from build123d import *

# Parameters (mm, degrees)
BOSS_EXTRUDE1_DEPTH = 9
FILLET1_R           = 6
FILLET2_R           = 4
BOSS_EXTRUDE2_DEPTH = 18
LPATTERN1_COUNT     = 6
LPATTERN1_PITCH     = 6
CUT_EXTRUDE1_DEPTH  = 26
CUT_EXTRUDE3_DEPTH  = 10
SKETCH5_R           = 1.5
CUT_EXTRUDE4_DEPTH  = 124.909348227
SKETCH6_R           = 1.75
BOSS_EXTRUDE3_DEPTH = 3
SKETCH7_R           = 1.25
CUT_EXTRUDE6_DEPTH  = 1
SKETCH8_R           = 1.25
CUT_EXTRUDE7_DEPTH  = 1
CUT_EXTRUDE8_DEPTH  = 1


with BuildPart() as part:
    # Sketch1 → Boss-Extrude1 (new, symmetric)
    with BuildSketch(Plane(origin=(0, 0, 0), x_dir=(1, 0, 0), z_dir=(0, 1, 0))):
        with BuildLine():
            ThreePointArc((13.432245527, -50.487906924), (21.509028276, -53.088979862), (18.907955338, -61.165762611))
            Line((18.907955338, -61.165762611), (11, -67.286566673))
            Line((11, -67.286566673), (11, -117.286566673))
            Line((11, -117.286566673), (0, -117.286566673))
            Line((0, -117.286566673), (0, -110.286566673))
            Line((0, -110.286566673), (-20.129396013, -88.042299634))
            Line((-20.129396013, -88.042299634), (-31.928362438, -82.58479184))
            Line((-31.928362438, -82.58479184), (-27.730279519, -73.508663821))
            Line((-27.730279519, -73.508663821), (-24.896421124, -73.027946621))
            Line((-24.896421124, -73.027946621), (-12.941547125, -71))
            Line((-12.941547125, -71), (-4.10711559, -69.126148868))
            Line((-4.10711559, -69.126148868), (13.432245527, -50.487906924))
        make_face()
        Polygon((-12.941547125, -71), (-24.896421124, -73.027946621), (-36.603518956, -4.013862114), (-12.941547125, 0), align=None)
    extrude(amount=BOSS_EXTRUDE1_DEPTH, both=True)

    # Fillet1
    fillet1_edges = [part.edges().sort_by_distance(p)[0] for p in [
        (-36.603518956, 0, 4.013862114),
        (-12.941547125, 0, 0),
    ]]
    fillet(fillet1_edges, radius=FILLET1_R)

    # Fillet2
    fillet2_edges = [part.edges().sort_by_distance(p)[0] for p in [
        (0, 0, 117.286566673),
        (-31.928362438, 0, 82.58479184),
        (-27.730279519, 0, 73.508663821),
    ]]
    fillet(fillet2_edges, radius=FILLET2_R)

    # Sketch2 → Boss-Extrude2 (add)
    with BuildSketch(Plane(origin=(0, 9, 0), x_dir=(1, 0, 0), z_dir=(0, 1, 0))):
        Polygon((15, -112.286566673), (11, -114.265571656), (11, -110.265571656), align=None)
    boss_extrude2 = extrude(amount=-BOSS_EXTRUDE2_DEPTH)

    # LPattern1: Boss-Extrude2 ×6
    with Locations(*[(0, 0, -i * LPATTERN1_PITCH) for i in range(1, LPATTERN1_COUNT)]):
        add(boss_extrude2)

    # Sketch3 → Cut-Extrude1 (cut)
    with BuildSketch(Plane(origin=(0, 9, 0), x_dir=(1, 0, 0), z_dir=(0, 1, 0))):
        Polygon((8.082911966, -112.457569416), (8.082911966, -87.457569416), (-6.917088034, -87.457569416), align=None)
    extrude(amount=-CUT_EXTRUDE1_DEPTH, mode=Mode.SUBTRACT)

    # Sketch4 → Cut-Extrude3 (cut)
    with BuildSketch(Plane(origin=(-54.869240858, 0, 49.65255435), x_dir=(0.6709798671072843, 0, 0.7414755679971466), z_dir=(-0.7414755679971466, 0, 0.6709798671072843))):
        Polygon((60.774794667, 6), (60.774794667, -6), (78.951118156, -8.019187605), (78.951118156, 8.019187605), align=None)
    extrude(amount=-CUT_EXTRUDE3_DEPTH, mode=Mode.SUBTRACT)

    # Sketch5 → Cut-Extrude4 (cut, through all)
    with BuildSketch(Plane(origin=(0, 9, 0), x_dir=(1, 0, 0), z_dir=(0, 1, 0))):
        with Locations(Location((-29.68456047, -8.925889543, 0), (0, 0, 270))):
            Circle(SKETCH5_R)
    extrude(amount=-CUT_EXTRUDE4_DEPTH, mode=Mode.SUBTRACT)

    # Sketch6 → Boss-Extrude3 (add)
    with BuildSketch(Plane(origin=(0, 9, 0), x_dir=(1, 0, 0), z_dir=(0, 1, 0))):
        with Locations(Location((-26.618678063, -80.6335738, 0), (0, 0, 270))):
            Circle(SKETCH6_R)
        with Locations(Location((16.170100432, -55.826834767, 0), (0, 0, 270))):
            Circle(SKETCH6_R)
    boss_extrude3 = extrude(amount=BOSS_EXTRUDE3_DEPTH)

    # Sketch7 → Cut-Extrude6 (cut)
    with BuildSketch(Plane(origin=(0, 12, 0), x_dir=(1, 0, 0), z_dir=(0, 1, 0))):
        with Locations(Location((-26.618678063, -80.6335738, 0), (0, 0, 270))):
            Circle(SKETCH7_R)
    extrude(amount=-CUT_EXTRUDE6_DEPTH, mode=Mode.SUBTRACT)

    # Sketch8 → Cut-Extrude7 (cut)
    with BuildSketch(Plane(origin=(0, 12, 0), x_dir=(1, 0, 0), z_dir=(0, 1, 0))):
        with Locations(Location((16.170100432, -55.826834767, 0), (0, 0, 270))):
            Circle(SKETCH8_R)
    extrude(amount=-CUT_EXTRUDE7_DEPTH, mode=Mode.SUBTRACT)

    # Sketch9 → Cut-Extrude8 (cut)
    with BuildSketch(Plane(origin=(0, 9, 0), x_dir=(1, 0, 0), z_dir=(0, 1, 0))):
        with BuildLine():
            Line((-25.196199852, -15.539852581), (-16.757464085, -65.251677823))
            ThreePointArc((-16.757464085, -65.251677823), (-19.027845143, -68.450467492), (-22.226634811, -66.180086434))
            Line((-22.226634811, -66.180086434), (-30.665370577, -16.468261192))
            ThreePointArc((-30.665370577, -16.468261192), (-28.39498952, -13.269471524), (-25.196199852, -15.539852581))
        make_face()
    cut_extrude8 = extrude(amount=-CUT_EXTRUDE8_DEPTH, mode=Mode.SUBTRACT)

    # Mirror1: Boss-Extrude3, Cut-Extrude8 across plane
    add(boss_extrude3.mirror(Plane.ZX))
    add(cut_extrude8.mirror(Plane.ZX), mode=Mode.SUBTRACT)


solid = part.part
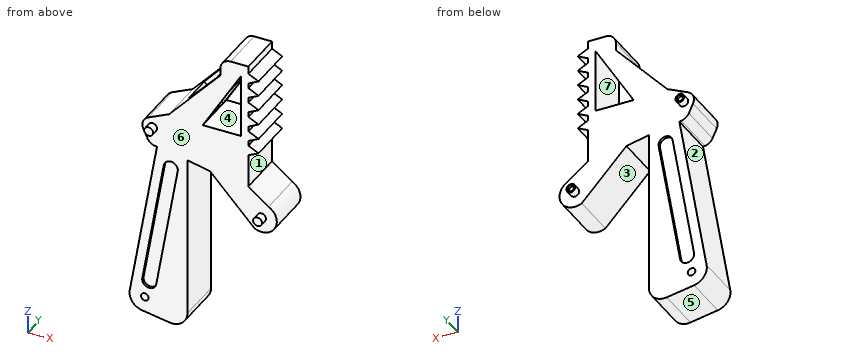
Model file for the job. Use its own axes, mm. Face numbers are marked on the shaded views. A direction names the side the tool comes from. Round coordinates to 2 decimals unless told otherwise and drop trailing zeros. Loops run counter-clockwise (first coordinate to the right, second up) from the corner with the lowest first, then second, coordinate; pieces in that order, holes last. Notation, with made-up numbers: (26.5, 63.25) -> (37.5, 63.25) arc R7 cw to (37.5, 73.25) -> close; hole circle Ø2 at (2.25, 56.25). An arc over 180 degrees is marked (long way). Answer as CSV lines item,"result". Start each with the question number.
1) Slice it at C-C (y = -10.25). List the corners of the cut face in (x, z), plus the area to 3 significant figures.
2) Probe line 1 along X through (y, z) = (8.5, 48); line 2 along Z through (x, y) = (7, 2.5); line 3 along Y through (x, z) = (-15.5, 22). List the from-to ranges inside material, lowest first.
3) Pin check, flat tips, straight feed: P1, Ø7.5, axis at x = -0.5, y = -4.5, coming from the +Z side; P2, Ø3, axis at x = -4, z = 87.5, coming from the +Y side; P3, Ø0.8, axis at x = -26.5, z = 81, coming from the +Y side. Stop position of each tip, or through.
4) Slice it at D-D (x = -11.5). List the corners of the cut face in (y, z).
5) Tool access for the marked faces 1, 2 and 3: list every direction of +Z, -Z, +X, -X, +Y, -Y with a clear straight run to the whole face (end or side of a thin tool).
6) Mould opens along X. For the marked faces 4, 5, 6 and 7 say: +X half, -X half, draft (parallel to the pull), parting line (faces both ways), or undercut.
7) Slice it at B-B (x = 6). List the corners of the cut face in (y, z), plus the area to 3 significant figures.
8) Slice it at A-A (z = 52). List the corners of the cut face in (x, y).
Filled in:
1,outline,"circle Ø3.5 at (-26.62, 80.63); circle Ø3.5 at (16.17, 55.83)"
1,area,"19.2 mm2"
2,line 1,"x = -29.14 to -25.31, -19.69 to -12.94"
2,line 2,"z = 57.32 to 87.46, 110.65 to 117.29"
2,line 3,"y = -9 to 9"
3,P1,"stops at z = 117.22"
3,P2,"stops at y = 9"
3,P3,"stops at y = 11"
4,outline,"(-9, 70.69) -> (9, 70.69) -> (9, 97.58) -> (6.43, 97.58) -> (6, 92.37) -> (-6, 92.37) -> (-6.43, 97.58) -> (-9, 97.58) -> close"
5,face 1,"+X, +Y, -Y"
5,face 2,"-X, +Y, -Y"
5,face 3,"-Z, +Y, -Y"
6,face 4,"undercut"
6,face 5,"-X half"
6,face 6,"draft"
6,face 7,"undercut"
7,outline,"(-9, 58.39) -> (9, 58.39) -> (9, 87.46) -> (-9, 87.46) -> close; (-9, 108.99) -> (9, 108.99) -> (9, 117.29) -> (-9, 117.29) -> close"
7,area,"673 mm2"
8,outline,"(-28.46, -9) -> (-24.63, -9) -> (-24.63, -8) -> (-19.01, -8) -> (-19.01, -9) -> (-12.94, -9) -> (-12.94, 9) -> (-19.01, 9) -> (-19.01, 8) -> (-24.63, 8) -> (-24.63, 9) -> (-28.46, 9) -> close; (12.01, -9) -> (20.79, -9) -> (20.79, 9) -> (12.01, 9) -> close"
